Part model, mm, in its own coordinate system. A direction names the side the tool comes from. Round coordinates to 2 decimals unless told otherwise and drop trailing zeros. Loops run counter-clockwise (first coordinate to the right, second up) from the corner with the lowest first, then second, coordinate; pieces in that order, holes last.
from build123d import *

# Parameters (mm, degrees)
F3_R     = 10
F4_DEPTH = 873.001


with BuildPart() as f1:
    # F0 (on Front) → F1 (revolve)
    with BuildSketch(Plane.XZ):
        Polygon((408.5, 109.5), (0, 109.5), (0, 101), (436.5, 101), (436.5, 172), (408.5, 172), align=None)
    revolve(axis=Axis((75.477585, 0, 0), (1, 0, 0)))

    # F2: F1 across plane


with BuildPart() as f1_1:
    add(f1.part)
    add(f1.part.mirror(Plane.YZ))

    # F3 (on face) → F4 (cut, through all)
    with BuildSketch(Plane.YZ.offset(436.5)):
        with Locations((0, 152)):
            Circle(F3_R)
    extrude(amount=-F4_DEPTH, mode=Mode.SUBTRACT)


solid = f1_1.part
1) Tool access for faces 5 (the face through (-436.5, 74, -74)), 6 (the face through (5.719, 106.896, -23.737)): list every direction of +Z, -Z, +X, -X, +Y, -Y with a clear straight run to the whole face (end or side of a thin tool).
Values:
face 5: +Z, -Z, -X, +Y, -Y
face 6: none
2) Wall check: line 1 along Z through (x, y) = (422, 0); line 2 along Z through (x, y) = (105, 0); line 3 along X through (y, z) = (141.5, 72). Give the ranges that are in metal, low to high.
Values:
line 1: z = -172 to -101, 101 to 142, 162 to 172
line 2: z = -109.5 to -101, 101 to 109.5
line 3: x = -436.5 to -408.5, 408.5 to 436.5
3) Slice it at C-C, the plane y = -130. Give the cut face in (x, z), then the cut area to 3 significant figures.
Values:
outline: (-436.5, -112.62) - (-408.5, -112.62) - (-408.5, 112.62) - (-436.5, 112.62) - close; (408.5, -112.62) - (436.5, -112.62) - (436.5, 112.62) - (408.5, 112.62) - close
area: 12,600 mm2
4) Slice it at B-B, the plane y = 0. Give the cut face in (x, z).
Values:
outline: (-436.5, -172) - (-408.5, -172) - (-408.5, -109.5) - (408.5, -109.5) - (408.5, -172) - (436.5, -172) - (436.5, -101) - (-436.5, -101) - close; (-436.5, 101) - (436.5, 101) - (436.5, 142) - (408.5, 142) - (408.5, 109.5) - (-408.5, 109.5) - (-408.5, 142) - (-436.5, 142) - close; (-436.5, 162) - (-408.5, 162) - (-408.5, 172) - (-436.5, 172) - close; (408.5, 162) - (436.5, 162) - (436.5, 172) - (408.5, 172) - close
5) Slice it at A-A, the plane z = 0. Give the cut face in (x, y).
Values:
outline: (-436.5, -172) - (-408.5, -172) - (-408.5, -109.5) - (408.5, -109.5) - (408.5, -172) - (436.5, -172) - (436.5, -101) - (-436.5, -101) - close; (-436.5, 101) - (436.5, 101) - (436.5, 172) - (408.5, 172) - (408.5, 109.5) - (-408.5, 109.5) - (-408.5, 172) - (-436.5, 172) - close
6) Drop flat-ended pins along their axis: pin 1 Ø1 at (x, y) = (-232, -74.5) entering from +Z; pin 2 Ø1.5 at (x, y) = (-280.5, 77) entering from +Z; pin 3 Ø12 at (x, z) = (-288.5, 47.5) entering from -Y; pin 4 Ø12 at (y, z) = (0, 152) entering from +X. Give the stop position or say it passes through.
Values:
pin 1: stops at z = 80.71
pin 2: stops at z = 78.59
pin 3: stops at y = -101.33
pin 4: passes through
7) Mould opens along Z. For faces 1 (the face through (422.304, -170.536, -22.391)), 2 (the face through (422.7, -2.17, 142.24)), 3 (the face through (408.5, 112, -2)), 4 (the face through (-422.3, -2.17, 142.24)) say: released by +Z, released by -Z, zero draft, split by the parting line, or undercut.
Values:
face 1: split by the parting line
face 2: undercut
face 3: zero draft
face 4: undercut
8) Slice it at D-D, the plane x = 314.5. Give the cut face in (y, z).
Values:
outline: circle Ø219 at (0, 0); hole circle Ø202 at (0, 0)
